The listing builds one solid part. Answer for the finished solid, in the listing's coordinates (mm). A direction names the side the tool comes from. Coordinates: 2 decimals unless noted, no trailing zeros. Order: outer loops, then holes, each group sorted by start corner. A loop starts at its lowest first (then second) coordinate and runs counter-clockwise, first axis right, second up.
from build123d import *

# Parameters (mm, degrees)
SKETCH_W        = 225
SKETCH_H        = 150
PAD_DEPTH       = 10
SKETCH005_R     = 11.5
POCKET_DEPTH    = 6
COPYSKETCH006_R = 3.2
POCKET001_DEPTH = 10
SKETCH006_R     = 16.5
POCKET002_DEPTH = 1.8
SKETCH007_R     = 52
POCKET003_DEPTH = 8
SKETCH008_W     = 23.96291
SKETCH008_H     = 15
POCKET004_DEPTH = 8


with BuildPart() as part:
    # Sketch → Pad (new body)
    with BuildSketch(Plane.XY):
        with Locations((112.5, 75)):
            Rectangle(SKETCH_W, SKETCH_H)
    extrude(amount=PAD_DEPTH)

    # Sketch005 → Pocket (cut)
    with BuildSketch(Plane(origin=(0, 0, 0), x_dir=(1, 0, 0), z_dir=(0, 0, -1))):
        with Locations((140, -42)):
            Circle(SKETCH005_R)
        with Locations((140, -108)):
            Circle(SKETCH005_R)
    extrude(amount=-POCKET_DEPTH, mode=Mode.SUBTRACT)

    # CopySketch006 → Pocket001 (cut)
    with BuildSketch(Plane(origin=(0, 0, 0), x_dir=(1, 0, 0), z_dir=(0, 0, -1))):
        with Locations((140, -42)):
            Circle(COPYSKETCH006_R)
        with Locations((140, -108)):
            Circle(COPYSKETCH006_R)
    extrude(amount=-POCKET001_DEPTH, mode=Mode.SUBTRACT)

    # Sketch006 (on Face4 of Pocket001) → Pocket002 (cut)
    with BuildSketch(Plane(origin=(0, 0, 0), x_dir=(1, 0, 0), z_dir=(0, 0, -1))):
        with Locations((25, -25)):
            Circle(SKETCH006_R)
        with Locations((25, -125)):
            Circle(SKETCH006_R)
        with Locations((200, -25)):
            Circle(SKETCH006_R)
        with Locations((200, -125)):
            Circle(SKETCH006_R)
    extrude(amount=-POCKET002_DEPTH, mode=Mode.SUBTRACT)

    # Sketch007 (on Face5 of Pocket002) → Pocket003 (cut)
    with BuildSketch(Plane.XY.offset(10)):
        with Locations((75, 75)):
            Circle(SKETCH007_R)
    extrude(amount=-POCKET003_DEPTH, mode=Mode.SUBTRACT)

    # Sketch008 (on Face5 of Pocket003) → Pocket004 (cut)
    with BuildSketch(Plane.XY.offset(10)):
        with Locations((11.981453, 75)):
            Rectangle(SKETCH008_W, SKETCH008_H)
    extrude(amount=-POCKET004_DEPTH, mode=Mode.SUBTRACT)


solid = part.part
1) A tool of negligible diameter and unlimited length cuts with its end or side. For faces 1 (the face through (111, 0, 5)), 2 (the face through (183.516, 24.275, 0.887)), 3 (the face through (77, 76, 2)), from which of +Z, -Z, +X, -X, +Y, -Y can it reach the whole face along a straight path? Write none if from no direction.
2) Section B-B (z = 4) is taken. Give the vertices of the cut face in (x, y), then the cut area to 3 significant figures.
3) Each of these flat-tipped pins is pushed along its axis until it touches: P1, Ø16.5, axis at x = 194.5, y = 28.5, coming from the -Z side; P2, Ø1, axis at x = 51.5, y = 54, coming from the +Z side; P3, Ø1, axis at y = 78.5, z = 6.5, coming from the -X side. Where does it stop, or does it pass through?
4) Consider L1, parallel to Y at x = 25, z = 0.85; L2, parallel to X at y = 116, z = 5.75; L3, parallel to Y at x = 39, z = 9.75. Determine where each line is inside the solid, lowest interval first.
5) Section C-C (x = 200) is taken. Give the vertices of the cut face in (y, z).
6) Section A-A (x = 140) is taken. Give the vertices of the cut face in (y, z), then the cut area to 3 significant figures.
7) Section D-D (y = 64.5) is taken. Give the vertices of the cut face in (x, z), then the cut area to 3 significant figures.
8) Determine the mould class of faces 4 (the face through (12, 82.5, 6)), 5 (the face through (225, 74, 5)), 6 (the face through (111, 150, 5)) for opening direction Y: released by +Y, released by -Y, zero draft, split by the parting line, or undercut.
Filled sheet:
1. face 1: +Z, -Z, +X, -X, -Y
1. face 2: -Z
1. face 3: +Z
2. outline: (0, 0) - (225, 0) - (225, 150) - (0, 150) - (0, 82.5) - (23.54, 82.5) arc R52 cw (long way) to (23.54, 67.5) - (0, 67.5) - close; hole circle Ø23 at (140, 42); hole circle Ø23 at (140, 108)
2. area: 24,100 mm2
3. P1: stops at z = 1.8
3. P2: stops at z = 2
3. P3: stops at x = 126.85
4. L1: y = 0 to 8.5, 41.5 to 108.5, 141.5 to 150
4. L2: x = 0 to 43.02, 106.98 to 131.74, 148.26 to 225
4. L3: y = 0 to 37.48, 112.52 to 150
5. outline: (0, 0) - (8.5, 0) - (8.5, 1.8) - (41.5, 1.8) - (41.5, 0) - (108.5, 0) - (108.5, 1.8) - (141.5, 1.8) - (141.5, 0) - (150, 0) - (150, 10) - (0, 10) - close
6. outline: (0, 0) - (30.5, 0) - (30.5, 6) - (38.8, 6) - (38.8, 10) - (0, 10) - close; (45.2, 6) - (53.5, 6) - (53.5, 0) - (96.5, 0) - (96.5, 6) - (104.8, 6) - (104.8, 10) - (45.2, 10) - close; (111.2, 6) - (119.5, 6) - (119.5, 0) - (150, 0) - (150, 10) - (111.2, 10) - close
6. area: 1,170 mm2
7. outline: (0, 0) - (225, 0) - (225, 10) - (125.93, 10) - (125.93, 2) - (24.07, 2) - (24.07, 10) - (0, 10) - close
7. area: 1,440 mm2
8. face 4: undercut
8. face 5: zero draft
8. face 6: released by +Y
